Here's the drawing with two shaded views (mm, measured from the low corner). I have some questions. Coordinates: 2 decimals unless noted, no trailing zeros. Write each loop counter-clockwise with the first axis right and the second up, starting at its lowest first coordinate (ties: lowest second). Pieces come first, ordered by that corner, then holes. Notation, with made-up numbers: (-16, -30) - (1, -30) arc R25 cw to (1, -14) - close; hole circle Ø10 at (81, 64.5). An arc over 180 degrees is marked (long way). Answer in a Markdown table with one row per item. Add a question column.
Item 1: I'm going to push a flat-ended pin straight in: pin 1 (0.8 mm diameter, centred on x = 2.5, y = 0.5, fed in from +Z). Where does the tip first touch, or does it pass through?
Item 2: Imagine slicing it at A-A (z = 2.75). Please give me the cut outline in (x, y), plus the area to 3 significant figures.
Item 3: Imagine slicing it at C-C (y = 0.5). Please give me the cut outline in (x, z), plus the area to 3 significant figures.
Item 4: Imagine slicing it at B-B (x = 26.5). Please give me the cut outline in (y, z).
Item 5: Imagine slicing it at D-D (z = 19). Please give me the cut outline in (x, y), plus the area to 3 significant figures.
Item 6: If I drill on probe 1 along Z at (x, y) = (26.5, 0.6); probe 2 along X at (y, z) = (1.25, 8.5); probe 3 along X at (y, z) = (0.8, 2), over which ranges is the centre line in solid material (lowest first)? Write a range as from..to.
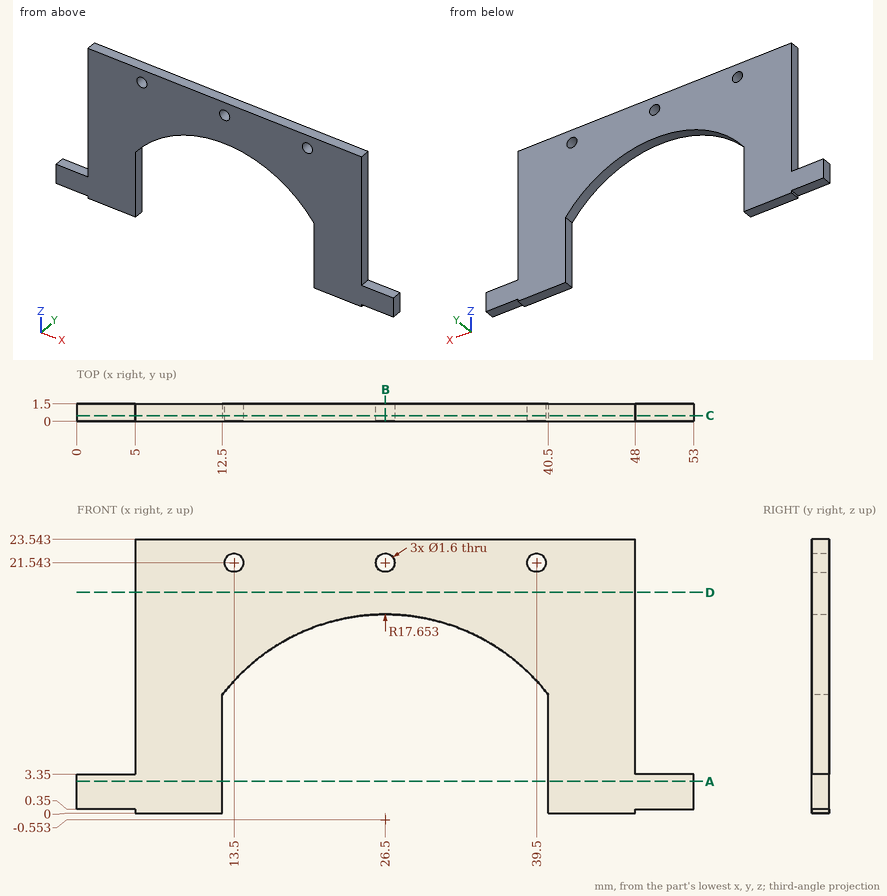
Here are the results:
| question | item | result |
|---|---|---|
| 1 | pin 1 | stops at z = 3.35 |
| 2 | outline | (0, 0) - (12.5, 0) - (12.5, 1.5) - (0, 1.5) - close; (40.5, 0) - (53, 0) - (53, 1.5) - (40.5, 1.5) - close |
| 2 | area | 37.5 mm2 |
| 3 | outline | (0, 0.35) - (5, 0.35) - (5, 0) - (12.5, 0) - (12.5, 10.2) arc R17.65 cw to (40.5, 10.2) - (40.5, 0) - (48, 0) - (48, 0.35) - (53, 0.35) - (53, 3.35) - (48, 3.35) - (48, 23.54) - (5, 23.54) - (5, 3.35) - (0, 3.35) - close; hole circle Ø1.6 at (13.5, 21.54); hole circle Ø1.6 at (26.5, 21.54); hole circle Ø1.6 at (39.5, 21.54) |
| 3 | area | 616 mm2 |
| 4 | outline | (0, 17.1) - (1.5, 17.1) - (1.5, 20.74) - (0, 20.74) - close; (0, 22.34) - (1.5, 22.34) - (1.5, 23.54) - (0, 23.54) - close |
| 5 | outline | (5, 0) - (48, 0) - (48, 1.5) - (5, 1.5) - close |
| 5 | area | 64.5 mm2 |
| 6 | probe 1 | z = 17.1..20.74, 22.34..23.54 |
| 6 | probe 2 | x = 5..12.5, 40.5..48 |
| 6 | probe 3 | x = 0..12.5, 40.5..53 |
